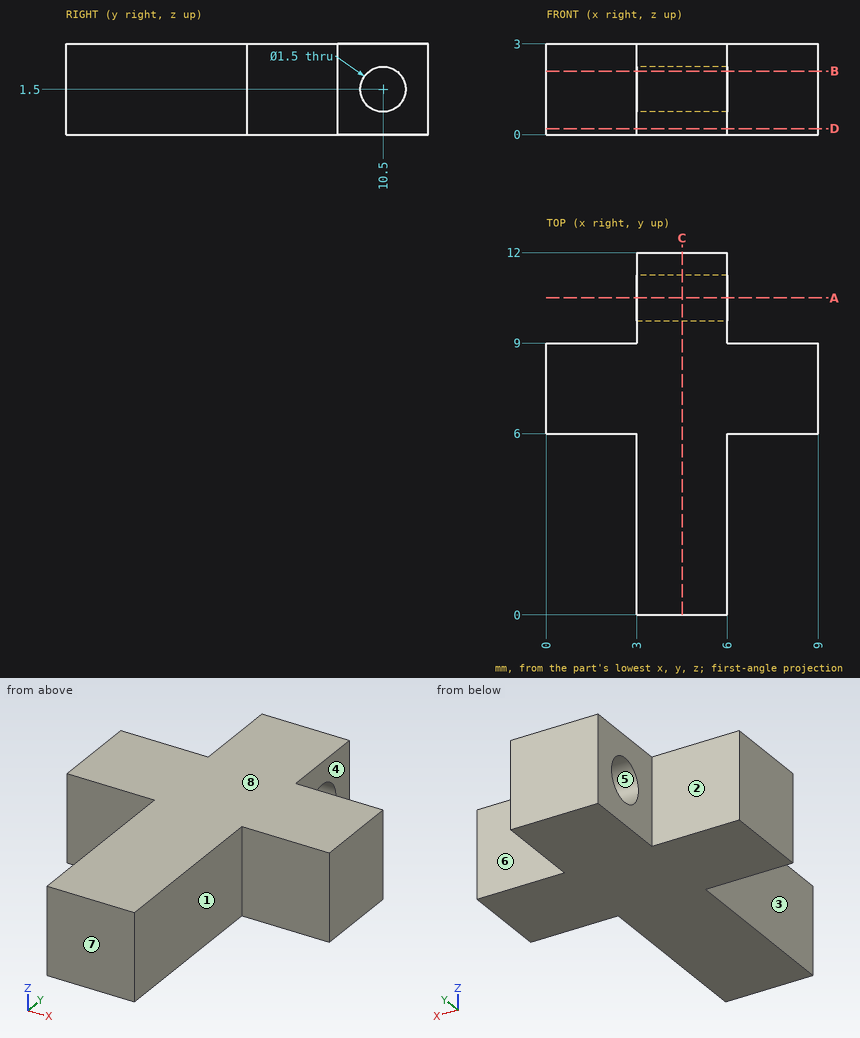
For this review, use the dimensioned drawing (mm, ordinates from the lowest corner) and the shaded views. A direction names the side the tool comes from. Round coordinates to 2 decimals unless told otherwise and drop trailing zeros. Order: outer loops, then holes, each group sorted by start corner. A loop starts at its lowest first (then second) coordinate and runs counter-clockwise, first axis right, second up.
1) Clearance check with flat-ended pins moving along their axes: pin 1 Ø0.9 at (y, z) = (11, 1) entering from +X; pin 2 Ø0.9 at (y, z) = (4, 1) entering from -X; pin 3 Ø1.5 at (x, z) = (1.5, 1) entering from -Y; pin 4 Ø1.2 at (y, z) = (10.5, 1.5) entering from -X. State where each tip first meets the part, or that it passes through.
The answers:
pin 1: stops at x = 6
pin 2: stops at x = 3
pin 3: stops at y = 6
pin 4: passes through
2) Draft analysis for pull direction Y (two halves, no side actions). For the marked faces 5, 6, 7 and 8, state which applies: released by +Y, released by -Y, zero draft, split by the parting line, or undercut.
The answers:
face 5: undercut
face 6: released by +Y
face 7: released by -Y
face 8: zero draft
3) Consider section A-A (y = 10.5). State the section outline as (x, z) points, plus the area to 3 significant figures.
The answers:
outline: (3, 0) - (6, 0) - (6, 0.75) - (3, 0.75) - close; (3, 2.25) - (6, 2.25) - (6, 3) - (3, 3) - close
area: 4.50 mm2
4) Machinability: for the marked faces 1, 2, 3 and 4, which of the approach directions +Z, -Z, +X, -X, +Y, -Y give a long, thin tool a straight path to every point of the face, cutting with its end or side? Answer none if there is none.
The answers:
face 1: +Z, -Z, +X, -Y
face 2: +Z, -Z, -X, +Y
face 3: +Z, -Z, -X, -Y
face 4: +Z, -Z, +X, +Y
5) Consider section C-C (x = 4.5). State the section outline as (y, z) points.
The answers:
outline: (0, 0) - (12, 0) - (12, 3) - (0, 3) - close; hole circle Ø1.5 at (10.5, 1.5)
6) Consider section B-B (z = 2.1). State the section outline as (x, y) points.
The answers:
outline: (0, 6) - (3, 6) - (3, 0) - (6, 0) - (6, 6) - (9, 6) - (9, 9) - (6, 9) - (6, 10.05) - (3, 10.05) - (3, 9) - (0, 9) - close; (3, 10.95) - (6, 10.95) - (6, 12) - (3, 12) - close
7) For L1, parallel to Z at x = 5.1, y = 10.5; L2, parallel to X at y = 0.75, z = 2.9; L3, parallel to Y at x = 7, z = 1.4, list the stretches that pass through material, from the lowest coordinate up.
The answers:
L1: z = 0 to 0.75, 2.25 to 3
L2: x = 3 to 6
L3: y = 6 to 9
8) Consider section D-D (z = 0.2). State the section outline as (x, y) points, plus the area to 3 significant figures.
The answers:
outline: (0, 6) - (3, 6) - (3, 0) - (6, 0) - (6, 6) - (9, 6) - (9, 9) - (6, 9) - (6, 12) - (3, 12) - (3, 9) - (0, 9) - close
area: 54.0 mm2
